```python
from build123d import *

# Parameters (mm, degrees)
F0_W      = 25
F0_H      = 25
F1_DEPTH  = 4
F2_W      = 25
F2_H      = 4
F3_DEPTH  = 20
F4_W      = 2
F4_H      = 20
F5_DEPTH  = 21
F6_SIZE2  = 20
F6_SIZE   = 21
F7_R      = 1.7
F8_DEPTH  = 25
F9_R      = 1.7
F10_DEPTH = 25


with BuildPart() as f1:
    # F0 (on Top) → F1 (new body)
    with BuildSketch(Plane.XY):
        with Locations((12.5, 12.5)):
            Rectangle(F0_W, F0_H)
    extrude(amount=F1_DEPTH)

    # F2 (on face) → F3 (join)
    with BuildSketch(Plane.XY.offset(4)):
        with Locations((12.5, 2)):
            Rectangle(F2_W, F2_H)
    extrude(amount=F3_DEPTH)

    # F4 (on face) → F5 (join)
    with BuildSketch(Plane(origin=(0, 4, 0), x_dir=(-1, 0, 0), z_dir=(0, 1, 0))):
        with Locations((-24, 14)):
            Rectangle(F4_W, F4_H)
        with Locations((-1, 14)):
            Rectangle(F4_W, F4_H)
    extrude(amount=F5_DEPTH)

    # F6
    f6_edges = [f1.edges().sort_by_distance(p)[0] for p in [
        (24, 25, 24),
        (1, 25, 24),
    ]]
    f6_side = f1.faces().sort_by_distance((0.353553, 12.5, 24))[0]
    chamfer(f6_edges, length=F6_SIZE, length2=F6_SIZE2, reference=f6_side)

    # F7 (on face) → F8 (cut)
    with BuildSketch(Plane(origin=(0, 4, 0), x_dir=(-1, 0, 0), z_dir=(0, 1, 0))):
        with Locations((-12.5, 14)):
            Circle(F7_R)
    extrude(amount=-F8_DEPTH, mode=Mode.SUBTRACT)

    # F9 (on face) → F10 (cut)
    with BuildSketch(Plane.XY.offset(4)):
        with Locations((12.5, 15)):
            Circle(F9_R)
    extrude(amount=-F10_DEPTH, mode=Mode.SUBTRACT)


solid = f1.part
```
Source: CAD feature listing. Evaluate the final solid. Frame: model axes, mm. A direction names the side the tool comes from. Round coordinates to 2 decimals unless told otherwise and drop trailing zeros. Order: outer loops, then holes, each group sorted by start corner. A loop starts at its lowest first (then second) coordinate and runs counter-clockwise, first axis right, second up. Notation, with made-up numbers: (-37.75, 23.5) -> (4.25, 23.5) arc R15 ccw to (4.25, 38.5) -> close; hole circle Ø3 at (-20.5, 7). An arc over 180 degrees is marked (long way). One line per item, written item: value. Start each with the question number.
Q1. Section query C-C (y = 2.5). Return the cut outline in (x, z).
Q2. Section query D-D (x = 17.5). Return the cut outline in (y, z), plus the area to 3 significant figures.
Q3. Pin query (flat end, axial travel): pin 1 (4 mm diameter, centred on x = 12.5, z = 14, fed in from +Y); pin 2 (1 mm diameter, centred on x = 7, y = 16, fed in from +Z). Return the tip coordinate at first contact, or that it passes through.
Q4. Section query B-B (x = 12.5). Return the cut outline in (y, z), plus the area to 3 significant figures.
Q5. Access query for faces 4 (the cylindrical face through (14.07, 14.35, 2.03)), 5 (the flat face through (23, 12, 12)). Directions: +Z, -Z, +X, -X, +Y, -Y. A direction counts if a zero-diameter tool reaches every point of the face in a straight line with its end or side. Return the directions, or none.
Q6. Section query A-A (z = 14). Return the cut outline in (x, y).
Q7. Material intervals for probe 1 along X at (y, z) = (11.25, 5); probe 2 along Z at (x, y) = (12.5, 0.9); probe 3 along Z at (x, y) = (2.5, 13.5), sorted ascending.
Q8. Draft query along X for faces 1 (the flat face through (13, 25, 2)), 2 (the flat face through (0, 10, 9)), 3 (the flat face through (12, 4, 16)). Return one class per face: pulls with the +X half, pulls with the -X half, needs draft (parallel to the pull), parting line crosses it, or undercut.
Findings below:
1. outline: (0, 0) -> (25, 0) -> (25, 24) -> (0, 24) -> close; hole circle Ø3.4 at (12.5, 14)
2. outline: (0, 0) -> (25, 0) -> (25, 4) -> (4, 4) -> (4, 24) -> (0, 24) -> close
2. area: 180 mm²
3. pin 1: y = 4
3. pin 2: z = 4
4. outline: (0, 0) -> (13.3, 0) -> (13.3, 4) -> (4, 4) -> (4, 12.3) -> (0, 12.3) -> close; (0, 15.7) -> (4, 15.7) -> (4, 24) -> (0, 24) -> close; (16.7, 0) -> (25, 0) -> (25, 4) -> (16.7, 4) -> close
4. area: 153 mm²
5. face 4: +Z, -Z
5. face 5: +Z, +Y
6. outline: (0, 0) -> (10.8, 0) -> (10.8, 4) -> (2, 4) -> (2, 14.5) -> (0, 14.5) -> close; (14.2, 0) -> (25, 0) -> (25, 14.5) -> (23, 14.5) -> (23, 4) -> (14.2, 4) -> close
7. probe 1: 0 to 2, 23 to 25
7. probe 2: 0 to 12.3, 15.7 to 24
7. probe 3: 0 to 4
8. face 1: needs draft
8. face 2: pulls with the -X half
8. face 3: undercut
